The listing builds one solid part. Answer for the finished solid, in the listing's coordinates (mm). A direction names the side the tool comes from. Give positions to 0.01 mm unless a question says otherwise; leave off trailing zeros. Order: outer loops, then holes, each group sorted by start corner. A loop starts at its lowest first (then second) coordinate and runs counter-clockwise, first axis right, second up. Notation, with made-up numbers: (38, 12) - (79, 12) arc R14 cw to (79, 35) - close; hole circle Ø9 at (62.25, -11.75). An arc over 180 degrees is marked (long way). Use a Markdown table: item, result. Add a question column.
1) Find section C-C, the plane x = 0.5. Determine the outline of the cut face in (y, z).
2) Flat-ended cylindrical pins translate along their axes: pin 1 (0.6 mm diameter, centred on x = 1.5, y = -1.5, fed in from +Z); pin 2 (1.3 mm diameter, centred on y = 1.5, z = 1.5, fed in from +X); pin 3 (1 mm diameter, centred on x = 1.5, z = 44, fed in from +Y); pin 4 (1.3 mm diameter, centred on x = 1.5, y = 1.5, fed in from +Z). Find the tip coordinate at first contact, or state that the pin passes through.
3) Find section B-B, the plane y = 1.75. Determine the outline of the cut face in (x, z), plus the area to 3 significant figures.
4) Find section A-A, the plane z = 19.5. Determine the outline of the cut face in (x, y), plus the area to 3 significant figures.
5) Straight lines are drawn through the part: line 1 (X direction, y = -0.1, z = 24.5); line 2 (Y direction, x = -1.3, z = 48.5); line 3 (Z direction, x = 1.35, y = -1.45). For each, find the intervals that lie inside material, in ascending order.
6) For faces 1 (the face through (-0.982, -2, 48)), 2 (the face through (-0.982, 2, 2)), 3 (the face through (-1.5, -1.5, 5)), 4 (the face through (0.982, 2, 2)), 5 (the face through (1.5, 1.4, 45)), determine the directions among +Z, -Z, +X, -X, +Y, -Y from which every point of the face is accessible in a straight line to the end or side of a thin tool.
Autodesk Fusion 360 part; units mm, degrees
sketch "Sketch1" plane through (0, 0, 0) normal (0, 0, 1) x (1, 0, 0)
  circle A0 centre (0, 0) radius 2.4
  dimension "d1" = 4.8
extrude "Extrude1" add sketch "Sketch1" along normal blind 50
sketch "Sketch2" plane through (0, 0, 50) normal (0, 0, 1) x (-1, 0, 0)
  circle A0 centre (0, 0) radius 2.4
  line L0 (0.9817, -0.9817) -> (-0.9817, -0.9817)
  line L1 (-0.9817, -0.9817) -> (-0.9817, 0.9817)
  line L2 (-0.9817, 0.9817) -> (0.9817, 0.9817)
  line L3 (0.9817, 0.9817) -> (0.9817, -0.9817)
  line L4 (0.9817, -0.9817) -> (-0.9817, 0.9817) construction
  line L5 (-0.9817, -0.9817) -> (0.9817, 0.9817) construction
  line L6 (0.9817, -0.9817) -> (2.1901, -0.9817)
  line L7 (0.9817, 0.9817) -> (2.1901, 0.9817)
  line L8 (-0.9817, 0.9817) -> (-2.1901, 0.9817)
  line L9 (-0.9817, -0.9817) -> (-2.1901, -0.9817)
  line L10 (-0.9817, -0.9817) -> (-0.9817, -2.1901)
  line L11 (0.9817, -0.9817) -> (0.9817, -2.1901)
  line L12 (0.9817, 0.9817) -> (0.9817, 2.1901)
  line L13 (-0.9817, 0.9817) -> (-0.9817, 2.1901)
extrude "Extrude2" cut sketch "Sketch2" against normal blind 5 contours A0 L7 L12 | A0 L6 L11 | A0 L8 L13 | A0 L9 L10
ref_plane "WorkPlane1" through (0, 0, 25) normal (0, 0, 1) x (1, 0, 0)
mirror "Mirror1" about plane through (0, 0, 25) normal (0, 0, 1) of "Extrude2"
The answers:
| question | item | result |
|---|---|---|
| 1 | outline | (-2.35, 0) - (2.35, 0) - (2.35, 50) - (-2.35, 50) - close |
| 2 | pin 1 | z = 45 |
| 2 | pin 2 | x = 2.24 |
| 2 | pin 3 | y = 2.18 |
| 2 | pin 4 | z = 50 |
| 3 | outline | (-1.64, 5) - (-0.98, 5) - (-0.98, 0) - (0.98, 0) - (0.98, 5) - (1.64, 5) - (1.64, 45) - (0.98, 45) - (0.98, 50) - (-0.98, 50) - (-0.98, 45) - (-1.64, 45) - close |
| 3 | area | 151 mm2 |
| 4 | outline | circle Ø4.8 at (0, 0) |
| 4 | area | 18.1 mm2 |
| 5 | line 1 | -2.4 to 2.4 |
| 5 | line 2 | -0.98 to 0.98 |
| 5 | line 3 | 5 to 45 |
| 6 | face 1 | +Z, -X, -Y |
| 6 | face 2 | -Z, -X, +Y |
| 6 | face 3 | -Z, -X, -Y |
| 6 | face 4 | -Z, +X, +Y |
| 6 | face 5 | +Z, +X, +Y |
